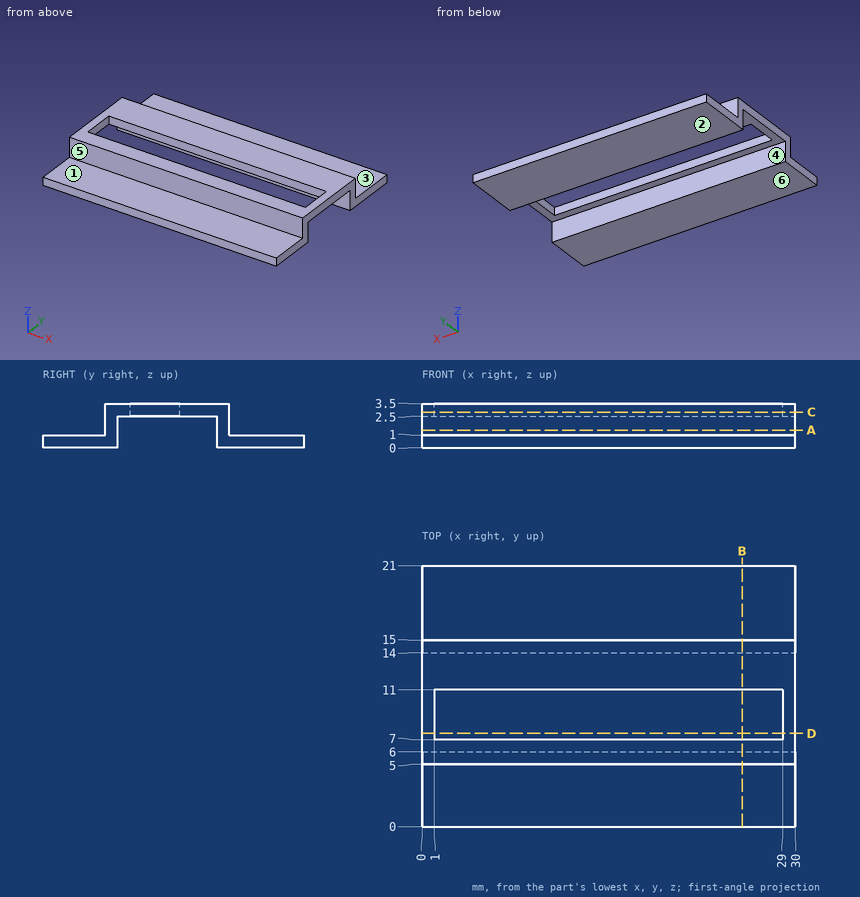
Verification items for this drawing (mm, ordinates from the low corner). A direction names the side the tool comes from. Give positions to 0.01 mm unless a question says otherwise; leave off trailing zeros. Loops run counter-clockwise (first coordinate to the right, second up) from the corner with the lowest first, then second, coordinate; pieces in that order, holes last. Notation, with made-up numbers: M 76,31.25 L 105,31.25 A23 ccw 105,67.25 Z; hole C 35,19.5 d8. An arc over 180 degrees is marked long. Return JSON: item names as keys, results as strings. Group by question number.
1. Mould release check, pull along Y, two halves, no side actions. Record for the marked faces 4, 5 and 6: released by +Y, released by -Y, zero draft, split by the parting line, or undercut.
2. Cross-section at D-D on y = 7.5. Record the boundary of the cut face in (x, z).
3. Cross-section at B-B on x = 25.75. Record the boundary of the cut face in (y, z).
4. Tool access check on the marked faces 1, 2 and 3. Record the directions out of +Z, -Z, +X, -X, +Y, -Y that give a thin tool (end or side, any length) a straight path to the whole face; none if there is none.
5. Cross-section at A-A on z = 1.4. Record the boundary of the cut face in (x, y), plus the area to 3 significant figures.
6. Go/stop test with flat-tipped pins: pin 1 (1.1 mm diameter, centred on x = 11.5, z = 3, fed in from +Y); pin 2 (3 mm diameter, centred on x = 4.5, y = 7, fed in from -Z); pin 3 (4 mm diameter, centred on x = 10.5, y = 10.5, fed in from -Z); pin 4 (1.5 mm diameter, centred on x = 3.5, z = 2.5, fed in from -Y). Record where each tip stops, or that it passes through.
7. Cross-section at C-C on z = 2.85. Record the boundary of the cut face in (x, y), plus the area to 3 significant figures.
8. Thickness scan on L1, parallel to Y at x = 25, z = 0.8; L2, parallel to Y at x = 26.5, z = 2.1; L3, parallel to Z at x = 11.5, y = 15.75. Record the ranges inside material, lowest first.
Return value:
{
 "1": {"face 4": "undercut", "face 5": "released by -Y", "face 6": "zero draft"},
 "2": {"outline": "M 0,2.5 L 1,2.5 L 1,3.5 L 0,3.5 Z; M 29,2.5 L 30,2.5 L 30,3.5 L 29,3.5 Z"},
 "3": {"outline": "M 0,0 L 6,0 L 6,2.5 L 7,2.5 L 7,3.5 L 5,3.5 L 5,1 L 0,1 Z; M 11,2.5 L 14,2.5 L 14,0 L 21,0 L 21,1 L 15,1 L 15,3.5 L 11,3.5 Z"},
 "4": {"face 1": "+Z, +X, -X, -Y", "face 2": "-Z, +X, -X, +Y, -Y", "face 3": "+Z, +X, -X, +Y"},
 "5": {"outline": "M 0,5 L 30,5 L 30,6 L 0,6 Z; M 0,14 L 30,14 L 30,15 L 0,15 Z", "area": "60.0 mm^2"},
 "6": {"pin 1": "y = 15", "pin 2": "z = 0", "pin 3": "z = 2.5", "pin 4": "y = 5"},
 "7": {"outline": "M 0,5 L 30,5 L 30,15 L 0,15 Z; hole M 1,7 L 29,7 L 29,11 L 1,11 Z", "area": "188 mm^2"},
 "8": {"L1": "0 to 6, 14 to 21", "L2": "5 to 6, 14 to 15", "L3": "0 to 1"}
}
